The listing builds one solid part. Answer for the finished solid, in the listing's coordinates (mm). A direction names the side the tool comes from. Coordinates: 2 decimals unless noted, no trailing zeros. Write each loop counter-clockwise with the first axis right and the second up, starting at its lowest first coordinate (ties: lowest second). Pieces come first, ordered by that corner, then holes.
Autodesk Inventor part; units mm, degrees
ref_plane "YZ Plane" through (0, 0, 0) normal (1, 0, 0) x (0, 1, 0)
ref_plane "XZ Plane" through (0, 0, 0) normal (0, 1, 0) x (-1, 0, 0)
ref_plane "XY Plane" through (0, 0, 0) normal (0, 0, 1) x (1, 0, 0)
sketch "Sketch1" plane through (0, 0, 0) normal (0, 1, 0) x (-1, 0, 0)
  line L0 (16.3, 12.25) -> (-16.3, 12.25)
  line L1 (-16.3, 12.25) -> (-16.3, -12.25)
  line L2 (-16.3, -12.25) -> (16.3, -12.25)
  line L3 (16.3, -12.25) -> (16.3, 12.25)
  line L4 (11.6, 11.6) -> (-11.6, 11.6)
  line L5 (-11.6, 11.6) -> (-11.6, -11.6)
  line L6 (-11.6, -11.6) -> (11.6, -11.6)
  line L7 (11.6, -11.6) -> (11.6, 11.6)
  point P0 (0, 0)
  point P1 (-11.6, 0)
  point P2 (-16.3, 0)
  point P3 (0, 12.25)
  point P4 (0, 11.6)
  dimension "d0" = 32.6
  dimension "d1" = 24.5
  dimension "d2" = 23.2
extrude "Extrusion1" add sketch "Sketch1" along normal blind 12 contours L3 L2 L1 L0 | L7 L6 L5 L4
extrude "Extrusion2" add sketch "Sketch1" against normal blind 4 contours L7 L6 L5 L4
sketch "Sketch2" plane through (0, -4, 0) normal (0, -1, 0) x (1, 0, 0)
  line L0 (11.6, 11.6) -> (-11.6, 11.6)
  line L1 (0, 11.6) -> (0, -11.6)
  line L2 (11.6, -11.6) -> (-11.6, -11.6)
  arc A0 (0, -11.6) -> (0, 11.6) centre (0, 0) ccw
revolve "Revolution1" add sketch "Sketch2" angle 360 about axis through (0, -4, 11.6) along (0, 0, -1)
properties part number "pir"
1. Section B-B on z = -1 is taken. Give the vertices of the cut face in (x, y), then the cut area to 3 significant figures.
Results found:
outline: (-16.3, 0) - (-11.6, 0) - (-11.6, -4) - (-11.56, -4) arc R11.56 ccw to (11.56, -4) - (11.6, -4) - (11.6, 0) - (16.3, 0) - (16.3, 12) - (-16.3, 12) - close
area: 694 mm2
2. Section D-D on x = 12 is taken. Give the vertices of the cut face in (y, z), then the cut area to 3 significant figures.
Results found:
outline: (0, -12.25) - (12, -12.25) - (12, 12.25) - (0, 12.25) - close
area: 294 mm2
3. A tool of negligible diameter and unlimited length cuts with its end or side. For faces 1 (the flat face through (0, -2, 11.6)), 2 (the flat face through (11.6, -2, 0)), 3 (the flat face through (9, -4, 9)), from which of +Z, -Z, +X, -X, +Y, -Y can it reach the whole face along a straight path? Write none if from no direction.
Results found:
face 1: +Z, +X, -X, -Y
face 2: +Z, -Z, +X, -Y
face 3: +Z, +X, -Y
4. Section C-C on y = -13 is taken. Give the vertices of the cut face in (x, z), then the cut area to 3 significant figures.
Results found:
outline: circle Ø14.64 at (0, 0)
area: 168 mm2
5. Section A-A on x = -5 is taken. Give the vertices of the cut face in (y, z).
Results found:
outline: (-4, -11.6) - (0, -11.6) - (0, -12.25) - (12, -12.25) - (12, 12.25) - (0, 12.25) - (0, 11.6) - (-4, 11.6) - (-4, 10.47) arc R10.47 ccw to (-4, -10.47) - close
6. Flat-ended cylindrical pins translate along their axes: P1, Ø1, axis at x = 4.5, y = -1, coming from the +Z side; P2, Ø2, axis at y = -10, z = 7, coming from the -X side; P3, Ø3, axis at y = -3, z = 5, coming from the -X side. Find the tip coordinate at first contact, or state that the pin passes through.
Results found:
P1: stops at z = 11.6
P2: stops at x = -8.19
P3: stops at x = -11.6
7. Find the intervals of material crossed by L1, parallel to Y at x = 12, z = 5.75; L2, parallel to X at y = -0.25, z = -5.75, in increasing order.
Results found:
L1: y = 0 to 12
L2: x = -11.6 to 11.6
